Check sheet for the modelled part. Datum: model origin and axes. Units: mm. A direction names the side the tool comes from. Give positions to 0.01 mm unless a question says otherwise; leave off trailing zeros. Order: outer loops, then holes, each group sorted by start corner. A loop starts at its lowest first (then second) coordinate and runs counter-clockwise, first axis right, second up. Notation, with made-up numbers: (16, 29) - (48, 29) arc R23 ccw to (48, 50) - close; hole circle Ø5 at (17.25, 26). An arc over 180 degrees is marked (long way). Answer in a Markdown table with one row per item.
Solid Edge part; units mm, degrees
sketch "Sketch1" plane through (0, 0, 0) normal (0, 0, 1) x (1, 0, 0)
  line L0 (16, -9) -> (0, -9)
  line L1 (0, 9) -> (16, 9)
  line L2 (16, 9) -> (16, -9)
  arc A0 (0, -9) -> (0, 9) centre (0, 0) cw
  circle A1 centre (0, 0) radius 5
extrude "Protrusion1" add sketch "Sketch1" along normal blind 18
hole "Furo_2" at (16, 0, 9) direction (-1, 0, 0) diameter 5 depth 16
hole "Furo_3" at (16, 0, 9) direction (-1, 0, 0) diameter 4.2 end up to next
(1) Cross-section at B-B, the plane z = 2.75. Record the cut outline in (x, y).
Geometry says:
| item | result |
|---|---|
| outline | (0, -9) - (16, -9) - (16, 9) - (0, 9) arc R9 ccw to start; hole circle Ø10 at (0, 0) |
(2) Gauge pin test, flat ends, axial feed: P1, Ø2, axis at x = 1, y = -3.5, coming from the +Z side; P2, Ø4, axis at x = -6, z = 7.5, coming from the +Y side; P3, Ø6, axis at y = 0, z = 9, coming from the +X side; P4, Ø6, axis at x = -4, z = 12, coming from the +Y side. Record the tip position at first contact, or that the pin passes through.
Geometry says:
| item | result |
|---|---|
| P1 | through |
| P2 | y = 8.06 |
| P3 | x = 16 |
| P4 | y = 8.94 |
(3) Cross-section at A-A, the plane y = 0. Record the cut outline in (x, z), then the cut area to 3 significant figures.
Geometry says:
| item | result |
|---|---|
| outline | (-9, 0) - (-5, 0) - (-5, 6.9) - (-9, 6.9) - close; (-9, 11.1) - (-5, 11.1) - (-5, 18) - (-9, 18) - close; (5, 0) - (16, 0) - (16, 6.5) - (5, 6.5) - close; (5, 11.5) - (16, 11.5) - (16, 18) - (5, 18) - close |
| area | 198 mm² |
(4) Thickness scan on L1, parallel to Z at x = 8.5, y = 0; L2, parallel to Y at x = 0.25, z = 16.25; L3, parallel to Z at x = -7.2, y = 0. Record the ranges inside material, lowest first.
Geometry says:
| item | result |
|---|---|
| L1 | 0 to 6.5, 11.5 to 18 |
| L2 | -9 to -4.99, 4.99 to 9 |
| L3 | 0 to 6.9, 11.1 to 18 |
(5) Mould release check, pull along Y, two halves, no side actions. Record for faces 1 (the cylindrical face through (-6.74, -0.8, 7.06)), 2 (the cylindrical face through (-4, 3, 9)), 3 (the flat face through (8, 9, 9)), 4 (the cylindrical face through (-8.39, -3.26, 8.87)): pulls with the +Y half, pulls with the -Y half, needs draft (parallel to the pull), parting line crosses it, or undercut.
Geometry says:
| item | result |
|---|---|
| face 1 | undercut |
| face 2 | undercut |
| face 3 | pulls with the +Y half |
| face 4 | parting line crosses it |
(6) Access from +Z, -Z, +X, -X, +Y, -Y to the whole of each face (thin tool, end or side, straight path). Record for faces 5 (the flat face through (6, 0, 18)), 6 (the cylindrical face through (10.1, -0.1, 11.5)).
Geometry says:
| item | result |
|---|---|
| face 5 | +Z, +X, -X, +Y, -Y |
| face 6 | +X |
(7) Cross-section at D-D, the plane x = -1.25. Record the cut outline in (y, z), then the cut area to 3 significant figures.
Geometry says:
| item | result |
|---|---|
| outline | (-8.91, 0) - (-4.84, 0) - (-4.84, 18) - (-8.91, 18) - close; (4.84, 0) - (8.91, 0) - (8.91, 18) - (4.84, 18) - close |
| area | 147 mm² |
(8) Cross-section at C-C, the plane x = 9. Record the cut outline in (y, z).
Geometry says:
| item | result |
|---|---|
| outline | (-9, 0) - (9, 0) - (9, 18) - (-9, 18) - close; hole circle Ø5 at (0, 9) |
